Could you check a few things on this model? Use its own coordinates, in mm. A direction names the side the tool comes from. Give positions to 0.01 mm unless a question says otherwise; leave off trailing zeros. Loops run counter-clockwise (first coordinate to the right, second up) from the corner with the lowest first, then second, coordinate; pieces in that order, holes last. Notation, with made-up numbers: (-31, 54.5) - (-18, 54.5) arc R15 cw to (-18, 59.5) - close; hole circle Ø7 at (29, 32.25). An arc over 180 degrees is marked (long way). Write each question's results on one line, items separated by ' | '. Start each with the question number.
```python
from build123d import *

# Parameters (mm, degrees)
BOSS_EXTRUDE1_DEPTH = 10
CUT_EXTRUDE1_DEPTH  = 62.373634991
SKETCH3_R           = 2
CUT_EXTRUDE2_DEPTH  = 3
CUT_EXTRUDE3_DEPTH  = 1.5
FILLET1_R           = 3
FILLET2_R           = 2


with BuildPart() as part:
    # Sketch1 → Boss-Extrude1 (new body)
    with BuildSketch(Plane(origin=(0, 0, 0), x_dir=(0, 0, -1), z_dir=(1, 0, 0))):
        Polygon((0, 0), (0, 45), (40.518181993, 0), align=None)
    extrude(amount=-BOSS_EXTRUDE1_DEPTH)

    # Sketch2 → Cut-Extrude1 (cut, through all)
    with BuildSketch(Plane(origin=(0, 0, 0), x_dir=(0, 0, -1), z_dir=(1, 0, 0))):
        Polygon((33.780071672, 3), (3, 37.184732806), (3, 3), align=None)
    extrude(amount=-CUT_EXTRUDE1_DEPTH, mode=Mode.SUBTRACT)

    # Sketch3 → Cut-Extrude2 (cut)
    with BuildSketch(Plane.XZ):
        with Locations(Location((-5, -8, 0), (0, 0, 270))):
            Circle(SKETCH3_R)
        with Locations(Location((-5, -23, 0), (0, 0, 270))):
            Circle(SKETCH3_R)
    extrude(amount=-CUT_EXTRUDE2_DEPTH, mode=Mode.SUBTRACT)

    # Sketch4 → Cut-Extrude3 (cut)
    with BuildSketch(Plane(origin=(0, 3, 0), x_dir=(1, 0, 0), z_dir=(0, 1, 0))):
        Polygon((-5, 19.1), (-1.622500925, 21.05), (-1.622500925, 24.95), (-5, 26.9), (-8.377499075, 24.95), (-8.377499075, 21.05), align=None)
        Polygon((-5, 11.9), (-8.377499075, 9.95), (-8.377499075, 6.05), (-5, 4.1), (-1.622500925, 6.05), (-1.622500925, 9.95), align=None)
    extrude(amount=-CUT_EXTRUDE3_DEPTH, mode=Mode.SUBTRACT)

    # Fillet1
    fillet1_edges = [part.edges().sort_by_distance(p)[0] for p in [
        (-5, 0, -40.518181993),
    ]]
    fillet(fillet1_edges, radius=FILLET1_R)

    # Fillet2
    fillet2_edges = [part.edges().sort_by_distance(p)[0] for p in [
        (-5, 3, -33.780071672),
    ]]
    fillet(fillet2_edges, radius=FILLET2_R)


solid = part.part
```
Q1. I want a section at A-A, the plane z = -23. List the corners of the cut face in (x, y) for me, then the cut area to 3 significant figures.
Q2. I want a section at C-C, the plane y = 13. List the corners of the cut face in (x, z) for me, then the cut area to 3 significant figures.
Q3. I'm going to push flat-ended pins straight in: pin 1 Ø3.5 at (x, z) = (-5, -8) entering from -Y; pin 2 Ø3 at (x, y) = (-4.5, 25.5) entering from -Z; pin 3 Ø3 at (x, z) = (-6, -10) entering from +Y. Where does each tip first touch, or does it pass through?
Q4. I want a section at B-B, the plane x = -3.5. List the corners of the cut face in (y, z) for me.
Q5. If we mould it in two halves opening along Z, with no side actions, what happens to faces 1 (the face through (0, 21, -18)), 2 (the face through (-5.07, 1.736, -36.501)), 3 (the face through (-5, 22, 0)), 4 (the face through (-8.377, 2, -23))? For each: +Z half, -Z half, draft (parallel to the pull), parting line (faces both ways), or undercut.
Q6. I want a section at D-D, the plane z = -13.5. List the corners of the cut face in (x, y) for me.
Q7. I need wall thicknesses on L1, parallel to X at y = 1, z = -23; L2, parallel to Z at x = -5, y = 19; L3, parallel to Z at x = -7.5, y = 21. Which ranges of each line are inside material? Lowest first, please. Write a range as from..to.
Q8. Which directions (+Z, -Z, +X, -X, +Y, -Y) give clear straight access to the entire face, cutting with the end or side of a thin tool? Please do faces 5 (the face through (-6.712, 2.26, -5.089)), 6 (the face through (-6.2, 0.7, -21.4)), 7 (the face through (-5.07, 4.157, -31.102)).
Conclusion:
1) outline: (-10, 0) - (-7, 0) - (-7, 1.5) - (-8.38, 1.5) - (-8.38, 3) - (-10, 3) - close; (-10, 14.97) - (0, 14.97) - (0, 19.46) - (-10, 19.46) - close; (-3, 0) - (0, 0) - (0, 3) - (-1.62, 3) - (-1.62, 1.5) - (-3, 1.5) - close | area: 58.7 mm^2
2) outline: (-10, -28.81) - (0, -28.81) - (0, -24.78) - (-10, -24.78) - close; (-10, -3) - (0, -3) - (0, 0) - (-10, 0) - close | area: 70.4 mm^2
3) pin 1: y = 29.69 | pin 2: z = -18.91 | pin 3: y = 35.56
4) outline: (0, -33.78) arc R3 ccw to (5.01, -36.01) - (45, 0) - (0, 0) - (0, -6.68) - (1.5, -6.68) - (1.5, -4.97) - (3, -4.97) - (3, -3) - (37.18, -3) - (6.34, -30.77) arc R2 cw to (3, -29.29) - (3, -26.03) - (1.5, -26.03) - (1.5, -24.32) - (0, -24.32) - close; (0, -21.68) - (1.5, -21.68) - (1.5, -19.97) - (3, -19.97) - (3, -11.03) - (1.5, -11.03) - (1.5, -9.32) - (0, -9.32) - close
5) face 1: draft | face 2: -Z half | face 3: +Z half | face 4: undercut
6) outline: (-10, 0) - (0, 0) - (0, 3) - (-10, 3) - close; (-10, 25.52) - (0, 25.52) - (0, 30.01) - (-10, 30.01) - close
7) L1: -10..-7, -3..0 | L2: -23.41..-19.37, -3..0 | L3: -21.61..-17.57, -3..0
8) face 5: none | face 6: -Y | face 7: +X, -X
